Geometry check sheet. Reference: the model listing, model coordinates, mm. A direction names the side the tool comes from. Give positions to 0.01 mm unless a question says otherwise; leave off trailing zeros. Write each loop counter-clockwise with the first axis right and the second up, starting at its lowest first coordinate (ties: lowest second). Pieces come first, ordered by that corner, then holes. Notation, with made-up numbers: (26, 85.25) - (78, 85.25) arc R31 cw to (78, 114.25) - close; hole circle Ø6 at (-24.75, 42). An arc over 180 degrees is marked (long way). One line per question, with ' | ' between items. Start each with the question number.
Q1. Section check B-B on y = 54. Record the boundary of the cut face in (x, z) (3 decimals), and give its area (3 significant figures).
Q2. Gauge pin test, flat ends, axial feed: P1, Ø4, axis at y = 21.5, z = 40, coming from the +X side; P2, Ø11.5, axis at x = 38.5, z = 27.5, coming from the -Y side; P3, Ø19.5, axis at y = -2, z = 6.5, coming from the +X side (3 decimals). Record the tip position at first contact, or that the pin passes through.
Q3. Section check A-A on z = 4. Record the boundary of the cut face in (x, y) (3 decimals).
Q4. Release check for a two-part mould opening along X. For faces 1 (the face through (22.225, 17, 20)), 2 (the face through (1, 7.938, 31)), 3 (the face through (109.945, -7.676, 52.575)) record: +X half, -X half, draft (parallel to the pull), parting line (faces both ways), or undercut.
Q5. Set-up check for faces 4 (the face through (32.727, 16.547, 54.785)), 5 (the face through (32.727, -16.791, 54.785)), 6 (the face through (86.569, 0.478, 66.674)): record each of +Z, -Z, +X, -X, +Y, -Y from which the full face is reachable in a straight line by a thin tool's end or side.
Q6. Thickness scan on L1, parallel to Y at x = 45.5, z = 54; L2, parallel to X at y = 1, z = -0.5 (3 decimals); L3, parallel to Y at x = 14.5, z = 39. Record the ranges inside material, lowest first. Write a range as [from, to].
```python
from build123d import *

# Parameters (mm, degrees)
F1_DEPTH = 63.5
F2_DEPTH = 25.4
F3_DEPTH = 7.9375
F5_R     = 5.08


with BuildPart() as f1:
    # F0 (on Front) → F1 (new body, symmetric)
    with BuildSketch(Plane.XZ):
        Polygon((-41.275, -9.525), (41.275, -9.525), (41.275, 9.525), (22.225, 9.525), (-41.275, 9.525), align=None)
    extrude(amount=F1_DEPTH, both=True)

    # F0 (on Front) → F2 (join, symmetric)
    with BuildSketch(Plane.XZ):
        with BuildLine():
            Line((22.225, 9.525), (41.275, 9.525))
            Line((41.275, 9.525), (41.275, 29.8189983006))
            ThreePointArc((41.275, 29.8189983006), (45.9246798487, 41.0443184519), (57.15, 45.6939983006))
            Line((57.15, 45.6939983006), (60.325, 45.6939983006))
            Line((60.325, 45.6939983006), (60.325, 64.7439983006))
            Line((60.325, 64.7439983006), (57.15, 64.7439983006))
            ThreePointArc((57.15, 64.7439983006), (32.4542956671, 54.5147026335), (22.225, 29.8189983006))
            Line((22.225, 29.8189983006), (22.225, 9.525))
        make_face()
    extrude(amount=F2_DEPTH, both=True)

    # F0 (on Front) → F3 (join, symmetric)
    with BuildSketch(Plane.XZ):
        with BuildLine():
            add(Edge.make_bspline(
                [(-41.275, 9.525), (-36.6270914674, 16.9778186828), (19.4735266268, 69.1415518522), (57.15, 64.7439983006)],
                knots=[0, 0, 0, 0, 112.8566276225, 112.8566276225, 112.8566276225, 112.8566276225], degree=3))
            Line((-41.275, 9.525), (22.225, 9.525))
            Line((22.225, 9.525), (22.225, 29.8189983006))
            ThreePointArc((22.225, 29.8189983006), (32.4542956671, 54.5147026335), (57.15, 64.7439983006))
        make_face()
    extrude(amount=F3_DEPTH, both=True)

    # F0 (on Front) → F4 (revolve)
    with BuildSketch(Plane.XZ):
        Polygon((85.416354239, 66.675), (85.6429753146, 45.6939983006), (85.725, 38.1), (111.125, 38.1), (111.125, 66.675), align=None)
    revolve(axis=Axis((85.5706771195, 0, 52.3875), (0.0108006215, 0, -0.9999416716)))

    # F5
    f5_edges = [f1.edges().sort_by_distance(p)[0] for p in [
        (41.275, -63.5, 0),
        (-41.275, -63.5, 0),
        (-41.275, 63.5, 0),
        (41.275, 63.5, 0),
    ]]
    fillet(f5_edges, radius=F5_R)


solid = f1.part
```
Working result:
1) outline: (-41.275, -9.525) - (41.275, -9.525) - (41.275, 9.525) - (-41.275, 9.525) - close | area: 1,570 mm2
2) P1: stops at x = 102.01 | P2: stops at y = -25.4 | P3: stops at x = 41.275
3) outline: (-41.275, -58.42) arc R5.08 ccw to (-36.195, -63.5) - (36.195, -63.5) arc R5.08 ccw to (41.275, -58.42) - (41.275, 58.42) arc R5.08 ccw to (36.195, 63.5) - (-36.195, 63.5) arc R5.08 ccw to (-41.275, 58.42) - close
4) face 1: -X half | face 2: draft | face 3: undercut
5) face 4: +Z, -X, +Y | face 5: +Z, -X, -Y | face 6: +Z, -X
6) L1: y = [-25.4, 25.4] | L2: x = [-41.275, 41.275] | L3: y = [-7.94, 7.94]
